Source: CAD feature listing. Evaluate the final solid. Frame: model axes, mm. Face numbers are marked on the shaded views. A direction names the side the tool comes from. Give positions to 0.01 mm unless a question says otherwise; leave off trailing zeros. Loops run counter-clockwise (first coordinate to the right, second up) from the corner with the lowest first, then second, coordinate; pieces in that order, holes last. Notation, with made-up numbers: M -2,-18 L 40,-18 A14 cw 40,-9 Z; hole C -14,39 d5. An arc over 180 degrees is marked long. Answer in a Markdown table with one row per item.
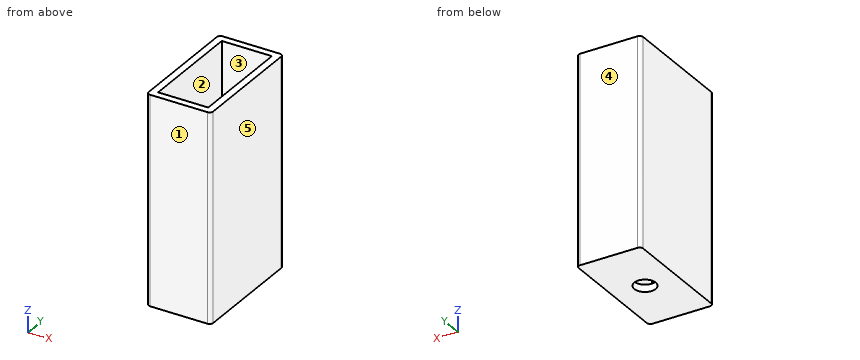
```python
from build123d import *

# Parameters (mm, degrees)
SKETCH_1_W          = 90
SKETCH_1_H          = 165
EXTRUDE_1_DEPTH     = 290
SHELL_1_T           = -10
FILLET_1_R          = 5
CUT_EXTRUDE_1_REACH = 347.579
SKETCH_2_R          = 15


with BuildPart() as part:
    # 스케치1 → 보스-돌출1 (new body)
    with BuildSketch(Plane.XY):
        with Locations((45, 82.5)):
            Rectangle(SKETCH_1_W, SKETCH_1_H)
    extrude(amount=EXTRUDE_1_DEPTH)

    # 쉘1
    shell_1_openings = [part.faces().sort_by_distance(p)[0] for p in [
        (45, 82.5, 290),
    ]]
    offset(amount=SHELL_1_T, openings=shell_1_openings, kind=Kind.INTERSECTION)

    # 필렛1
    fillet_1_edges = [part.edges().sort_by_distance(p)[0] for p in [
        (0, 165, 145),
        (90, 165, 145),
        (90, 0, 145),
        (0, 0, 145),
    ]]
    fillet(fillet_1_edges, radius=FILLET_1_R)

    # 스케치2 → 컷-돌출1 (cut, up to next)
    with BuildSketch(Plane(origin=(0, 0, 0), x_dir=(-1, 0, 0), z_dir=(0, 0, -1)), mode=Mode.PRIVATE) as cut_extrude_1_sk1:
        with Locations((-45, 82.5)):
            Circle(SKETCH_2_R)
    cut_extrude_1_tool1 = extrude(cut_extrude_1_sk1.sketch, amount=-CUT_EXTRUDE_1_REACH, mode=Mode.PRIVATE) & part.part
    add(cut_extrude_1_tool1.solids().sort_by_distance((45, 82.5, 0))[0], mode=Mode.SUBTRACT)


solid = part.part
```
Q1. Reachability of the marked faces 1 and 2 from +Z, -Z, +X, -X, +Y, -Y: full face, straight path, thin tool, end or side. Return the list, or none.
Values follow:
| item | result |
|---|---|
| face 1 | +Z, -Z, +X, -X, -Y |
| face 2 | +Z |
Q2. Ray query, probe 1 along Y at (x, z) = (45, 5); probe 2 along Y at (x, z) = (49.5, 74); probe 3 along X at (y, z) = (139.5, 231.5). Return the intervals inside material, ascending. Write a range as from..to.
Values follow:
| item | result |
|---|---|
| probe 1 | 0..67.5, 97.5..165 |
| probe 2 | 0..10, 155..165 |
| probe 3 | 0..10, 80..90 |
Q3. Section query A-A (y = 82.5). Output: boundary loops of the cut face in (x, z), plus the area to 3 significant figures.
Values follow:
| item | result |
|---|---|
| outline | M 0,0 L 30,0 L 30,10 L 10,10 L 10,290 L 0,290 Z; M 60,0 L 90,0 L 90,290 L 80,290 L 80,10 L 60,10 Z |
| area | 6,200 mm^2 |
Q4. Section query D-D (y = 104). Output: boundary loops of the cut face in (x, z).
Values follow:
| item | result |
|---|---|
| outline | M 0,0 L 90,0 L 90,290 L 80,290 L 80,10 L 10,10 L 10,290 L 0,290 Z |
Q5. Section query B-B (x = 45). Output: boundary loops of the cut face in (y, z), plus the area to 3 significant figures.
Values follow:
| item | result |
|---|---|
| outline | M 0,0 L 67.5,0 L 67.5,10 L 10,10 L 10,290 L 0,290 Z; M 97.5,0 L 165,0 L 165,290 L 155,290 L 155,10 L 97.5,10 Z |
| area | 6,950 mm^2 |
Q6. Mould query, pull axis Y, two halves, no side actions, for the marked faces 3, 4 and 5. Classes: +Y half, -Y half, draft (parallel to the pull), parting line (faces both ways), or undercut.
Values follow:
| item | result |
|---|---|
| face 3 | undercut |
| face 4 | +Y half |
| face 5 | draft |
Q7. Section query C-C (z = 39). Output: boundary loops of the cut face in (x, y).
Values follow:
| item | result |
|---|---|
| outline | M 0,5 A5 ccw 5,0 L 85,0 A5 ccw 90,5 L 90,160 A5 ccw 85,165 L 5,165 A5 ccw 0,160 Z; hole M 10,10 L 80,10 L 80,155 L 10,155 Z |
Q8. Contact query for a flat-ended pin moving along its axis: pin 1 Ø21 at (x, y) = (31.5, 70.5) entering from +Z. Output: stop coordinate, or through.
Values follow:
| item | result |
|---|---|
| pin 1 | z = 10 |
